Verification items for the finished model (mm, model axes). Round coordinates to 2 decimals unless told otherwise and drop trailing zeros. Write each loop counter-clockwise with the first axis right and the second up, starting at its lowest first coordinate (ties: lowest second). Pieces come first, ordered by that corner, then holes.
from build123d import *

# Parameters (mm, degrees)
SCHIZZO1_W                   = 2100
SCHIZZO1_H                   = 200
ESTRUSIONE_ESTRUSIONE1_DEPTH = 30
RACCORDO1_R                  = 15
SCHIZZO3_R                   = 7.5
ESTRUSIONE_ESTRUSIONE2_DEPTH = 30
RACCORDO2_R                  = 1
ESTRUSIONE_ESTRUSIONE3_START = 30
SCHIZZO4_R                   = 7.5
ESTRUSIONE_ESTRUSIONE3_DEPTH = 30
RACCORDO3_R                  = 1


with BuildPart() as part:
    # Schizzo1 → Estrusione-Estrusione1 (new body)
    with BuildSketch(Plane.XY):
        with Locations((1050, -100)):
            Rectangle(SCHIZZO1_W, SCHIZZO1_H)
    extrude(amount=ESTRUSIONE_ESTRUSIONE1_DEPTH)

    # Raccordo1
    raccordo1_edges = [part.edges().sort_by_distance(p)[0] for p in [
        (1050, 0, 0),
        (1050, 0, 30),
    ]]
    fillet(raccordo1_edges, radius=RACCORDO1_R - 0.0001)  # a hair under: the kernel refuses the full size

    # Schizzo3 → Estrusione-Estrusione2 (add)
    with BuildSketch(Plane(origin=(2100, 0, 0), x_dir=(0, 0, -1), z_dir=(1, 0, 0))):
        with Locations(Location((-15, -70, 0), (0, 0, 180))):
            Circle(SCHIZZO3_R)
        with Locations(Location((-15, -150, 0), (0, 0, 180))):
            Circle(SCHIZZO3_R)
    extrude(amount=ESTRUSIONE_ESTRUSIONE2_DEPTH)

    # Raccordo2
    raccordo2_edges = [part.edges().sort_by_distance(p)[0] for p in [
        (2130, -70, 7.5),
        (2130, -150, 7.5),
    ]]
    fillet(raccordo2_edges, radius=RACCORDO2_R)

    # Schizzo4 → Estrusione-Estrusione3 (add)
    with BuildSketch(Plane.ZY.offset(ESTRUSIONE_ESTRUSIONE3_START)):
        with Locations((15, -70)):
            Circle(SCHIZZO4_R)
        with Locations((15, -150)):
            Circle(SCHIZZO4_R)
    extrude(amount=-ESTRUSIONE_ESTRUSIONE3_DEPTH)

    # Raccordo3
    raccordo3_edges = [part.edges().sort_by_distance(p)[0] for p in [
        (-30, -70, 7.5),
        (-30, -150, 7.5),
    ]]
    fillet(raccordo3_edges, radius=RACCORDO3_R)


solid = part.part
Q1. Material ranges on line 1 along Y through (x, z) = (458, 16.5); line 2 along Y through (x, z) = (1880.5, 14); line 3 along X through (y, z) = (-136, 22.5), recorded low to high.
Recorded:
line 1: y = -200 to -0.08
line 2: y = -200 to -0.03
line 3: x = 0 to 2100
Q2. Depth check by flat-ended pin: P1, Ø10, axis at y = -137.5, z = 6, coming from the -X side; P2, Ø4, axis at y = -25, z = 11.5, coming from the +X side; P3, Ø1.5, axis at x = 1834, z = 9, coming from the +Y side. Enter the tip coordinate at first touch or a pass-through.
Recorded:
P1: stops at x = 0
P2: stops at x = 2100
P3: stops at y = -0.95
Q3. Sectioned sample at A-A (y = -118.5). Enter the section's corners in (x, z), plus the area to 3 significant figures.
Recorded:
outline: (0, 0) - (2100, 0) - (2100, 30) - (0, 30) - close
area: 63,000 mm2
